The model under review builds one solid part; all positions refer to its coordinate system, in mm. Face numbers are marked on the shaded views. Round coordinates to 2 decimals unless told otherwise and drop trailing zeros. Order: outer loops, then holes, each group sorted by start corner. A loop starts at its lowest first (then second) coordinate and runs counter-clockwise, first axis right, second up.
from build123d import *

# Parameters (mm, degrees)
F0_R      = 51.312695
F0_R_2    = 49.619791
F1_DEPTH  = 50
F2_R      = 51.280405
F3_DEPTH  = 5
F3_FACE_R = 51.280405
F4_DEPTH  = 5
F5_R      = 2.547455
F5_R_2    = 2.547454
F6_DEPTH  = 55.001


with BuildPart() as f1:
    # F0 (on Top) → F1 (new body)
    with BuildSketch(Plane.XY):
        Circle(F0_R)
        Circle(F0_R_2, mode=Mode.SUBTRACT)
    extrude(amount=-F1_DEPTH)

    # F2 (on Top) → F3 (join)
    with BuildSketch(Plane.XY):
        Circle(F2_R)
    extrude(amount=F3_DEPTH)

    # F3_face (on face) → F4 (join)
    with BuildSketch(Plane.XY.offset(5)):
        Circle(F3_FACE_R)
    extrude(amount=-F4_DEPTH)

    # F5 (on face) → F6 (cut, through all)
    with BuildSketch(Plane.XY.offset(5)):
        with Locations((-32.852452, 0)):
            Circle(F5_R)
        with Locations((28.030308, 0)):
            Circle(F5_R_2)
    extrude(amount=-F6_DEPTH, mode=Mode.SUBTRACT)


solid = f1.part
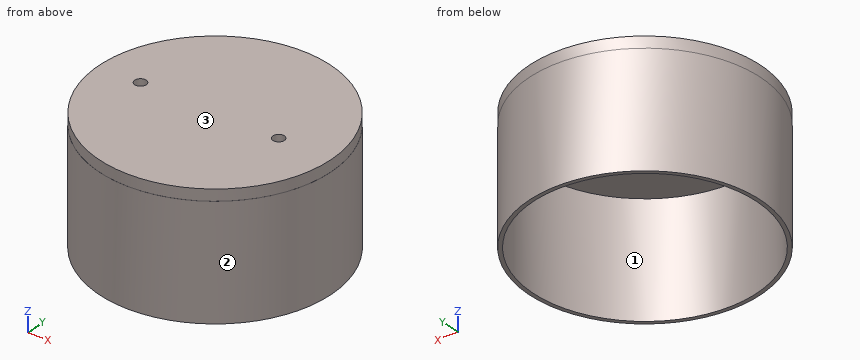
(1) We need section C-C (z = -7.5). Give the boundary of the cut face in (x, y).
(2) The part is to be moulded in two halves that separate along Y. For the marked faces 1, 2 and 3, say which applies: pulls with the +Y half, pulls with the -Y half, needs draft (parallel to the pull), parting line crosses it, or undercut.
(3) Clearance check with flat-ended pins moving along their axes: P1, Ø8, axis at x = 28.03, y = 0, coming from the -Z side; P2, Ø2, axis at x = 28, z = -40.5, coming from the -Y side; P3, Ø2, axis at y = -8.5, z = -7, coming from the +X side. State where each tip first meets the part, or that it passes through.
(4) To check wall thickness, follow L1, parallel to Y at x = 0, z = -11; L2, parallel to Z at x = 47, y = -5.5; L3, parallel to X at y = -32.5, z = -18. State the ranges of each line that lie inside material, in increasing order.
(5) We need section A-A (y = 0). Give the boundary of the cut face in (x, z) (3 decimals), and give its area (3 significant figures).
Verdict:
1. outline: circle Ø102.63 at (0, 0); hole circle Ø99.24 at (0, 0)
2. face 1: undercut
2. face 2: parting line crosses it
2. face 3: needs draft
3. P1: stops at z = 0
3. P2: stops at y = -43.63
3. P3: stops at x = 50.76
4. L1: y = -51.31 to -49.62, 49.62 to 51.31
4. L2: z = 0 to 5
4. L3: x = -39.71 to -37.49, 37.49 to 39.71
5. outline: (-51.313, -50) - (-49.62, -50) - (-49.62, 0) - (-35.4, 0) - (-35.4, 5) - (-51.28, 5) - (-51.28, 0) - (-51.313, 0) - close; (-30.305, 0) - (25.483, 0) - (25.483, 5) - (-30.305, 5) - close; (30.578, 0) - (49.62, 0) - (49.62, -50) - (51.313, -50) - (51.313, 0) - (51.28, 0) - (51.28, 5) - (30.578, 5) - close
5. area: 631 mm2
